```python
from build123d import *

# Parameters (mm, degrees)
SKETCH1_R                  = 12.7
BOSS_EXTRUDE1_DEPTH        = 15.875
SHELL1_T                   = -6.35
SKETCH4_R                  = 1.2446
CUT_EXTRUDE1_DEPTH         = 24.970724332
CUT_EXTRUDE1_DEPTH_BACK    = 24.970724332
SKETCH7_R                  = 7.6962
SKETCH7_R_2                = 6.35
CUT_EXTRUDE2_DEPTH         = 2.3622
TAP_DRILL_FOR_10_32_TAP1_D = 4.0386
CIRPATTERN1_COUNT          = 6


with BuildPart() as part:
    # Sketch1 → Boss-Extrude1 (new body)
    with BuildSketch(Plane.XY):
        Circle(SKETCH1_R)
    extrude(amount=-BOSS_EXTRUDE1_DEPTH)

    # Shell1
    shell1_openings = [part.faces().sort_by_distance(p)[0] for p in [
        (0, 0, -15.875),
    ]]
    offset(amount=SHELL1_T, openings=shell1_openings, kind=Kind.INTERSECTION)

    # Sketch4 → Cut-Extrude1 (cut, two sides)
    with BuildSketch(Plane(origin=(0, 0, 0), x_dir=(0, 0, -1), z_dir=(1, 0, 0))) as cut_extrude1_sk:
        with Locations((9.8425, 0)):
            Circle(SKETCH4_R)
    extrude(amount=CUT_EXTRUDE1_DEPTH, mode=Mode.SUBTRACT)
    extrude(cut_extrude1_sk.sketch, amount=-CUT_EXTRUDE1_DEPTH_BACK, mode=Mode.SUBTRACT)

    # Sketch7 → Cut-Extrude2 (cut)
    with BuildSketch(Plane(origin=(0, 0, -14.605), x_dir=(-1, 0, 0), z_dir=(0, 0, -1))):
        Circle(SKETCH7_R)
        with Locations(Location((0, 0, 0), (0, 0, 180))):
            Circle(SKETCH7_R_2, mode=Mode.SUBTRACT)
    extrude(amount=-CUT_EXTRUDE2_DEPTH, mode=Mode.SUBTRACT)

    # Tap Drill for #10-32 Tap1 (through all)
    with Locations(Plane.XY):
        with Locations((0, 0)):
            Hole(TAP_DRILL_FOR_10_32_TAP1_D / 2)

    # Sketch15 → Tap Drill for #4-40 Tap1 (revolve, cut)
    with BuildSketch(Plane(origin=(-10.16, 0, 0), x_dir=(0, -1, 0), z_dir=(1, 0, 0))):
        Polygon((0, 0), (0, 5.759152758), (1.1303, 5.08), (1.1303, 0), align=None)
    tap_drill_for_4_40_tap1 = revolve(axis=Axis((-10.16, 0, 6.35), (0, 0, -1)), mode=Mode.SUBTRACT)

    # CirPattern1: Tap Drill for #4-40 Tap1 ×6 about axis
    cirpattern1_axis = Axis((0, 0, 0), (0, 0, 1))
    for i in range(1, CIRPATTERN1_COUNT):
        add(tap_drill_for_4_40_tap1.rotate(cirpattern1_axis, i * 360 / CIRPATTERN1_COUNT), mode=Mode.SUBTRACT)


solid = part.part
```
Input: part model. Units: mm. Frame: model coordinates. A direction names the side the tool comes from. Round coordinates to 2 decimals unless told otherwise and drop trailing zeros. Order: outer loops, then holes, each group sorted by start corner. A loop starts at its lowest first (then second) coordinate and runs counter-clockwise, first axis right, second up. Notation, with made-up numbers: (42, -7.75) - (71, -7.75) arc R24 cw to (71, 2.25) - close; hole circle Ø10 at (37.5, 76.5). An arc over 180 degrees is marked (long way). Answer in a Markdown table with one row per item.
Item 1: Section query C-C (y = 5.5). Return the cut outline in (x, z) (3 decimals), then the cut area to 3 significant figures.
Model answer:
| item | result |
|---|---|
| outline | (-11.447, -15.875) - (-3.174, -15.875) - (-3.174, -14.605) - (-5.383, -14.605) - (-5.383, -12.243) - (-3.174, -12.243) - (-3.174, -6.35) - (3.174, -6.35) - (3.174, -12.243) - (5.383, -12.243) - (5.383, -14.605) - (3.174, -14.605) - (3.174, -15.875) - (11.447, -15.875) - (11.447, 0) - (-11.447, 0) - close |
| area | 293 mm² |
Item 2: Reachability of faces 4 (the cylindrical face through (-1.38, -6.2, -15.23)), 5 (the flat face through (0, -3, 0)), 6 (the cylindrical face through (9.057, -0.245, -2.504)), 7 (the flat face through (3, 6, -15.875)), 8 (the cylindrical face through (1.668, -7.513, -13.44)) from +Z, -Z, +X, -X, +Y, -Y: full face, straight path, thin tool, end or side. Return the list, or none.
Model answer:
| item | result |
|---|---|
| face 4 | -Z |
| face 5 | +Z, +X, -X, +Y, -Y |
| face 6 | +Z |
| face 7 | -Z, +X, -X, +Y, -Y |
| face 8 | none |
Item 3: Line query: line 1 (Y direction, x = 0, z = -14.05); line 2 (Z direction, x = -7.25, y = -1.75) (3 decimals); line 3 (X direction, y = 0.25, z = -12.5). Output: solid intervals per line, ascending.
Model answer:
| item | result |
|---|---|
| line 1 | y = -12.7 to -7.7, 7.7 to 12.7 |
| line 2 | z = -15.875 to -14.605, -12.243 to 0 |
| line 3 | x = -12.7 to -7.69, 7.69 to 12.7 |
Item 4: Section query B-B (z = -3). Return the cut outline in (x, y).
Model answer:
| item | result |
|---|---|
| outline | circle Ø25.4 at (0, 0); hole circle Ø2.26 at (-10.16, 0); hole circle Ø2.26 at (-5.08, -8.8); hole circle Ø2.26 at (-5.08, 8.8); hole circle Ø4.04 at (0, 0); hole circle Ø2.26 at (5.08, -8.8); hole circle Ø2.26 at (5.08, 8.8); hole circle Ø2.26 at (10.16, 0) |
Item 5: Pin query (flat end, axial travel): pin 1 (3 mm diameter, centred on x = 1.5, z = -5.5, fed in from -Y); pin 2 (6.5 mm diameter, centred on x = 0, y = 0, fed in from -Z); pin 3 (1 mm diameter, centred on y = -8, z = -2, fed in from +X); pin 4 (2 mm diameter, centred on x = -3, z = -6, fed in from -Y). Return the tip coordinate at first contact, or that it passes through.
Model answer:
| item | result |
|---|---|
| pin 1 | stops at y = -12.7 |
| pin 2 | stops at z = -6.35 |
| pin 3 | stops at x = 10.25 |
| pin 4 | stops at y = -12.54 |
Item 6: Section query A-A (x = 0). Return the cut outline in (y, z) (3 decimals), then the cut area to 3 significant figures.
Model answer:
| item | result |
|---|---|
| outline | (-12.7, -15.875) - (-6.35, -15.875) - (-6.35, -14.605) - (-7.696, -14.605) - (-7.696, -12.243) - (-6.35, -12.243) - (-6.35, -6.35) - (-2.019, -6.35) - (-2.019, 0) - (-12.7, 0) - close; (2.019, -6.35) - (6.35, -6.35) - (6.35, -12.243) - (7.696, -12.243) - (7.696, -14.605) - (6.35, -14.605) - (6.35, -15.875) - (12.7, -15.875) - (12.7, 0) - (2.019, 0) - close |
| area | 250 mm² |
Item 7: Mould query, pull axis Z, two halves, no side actions, for faces 1 (the conical face through (4.885, 8.824, -5.641)), 2 (the cylindrical face through (-6.083, -8.277, -2.504)), 3 (the cylindrical face through (-9.4, 0.1, -8.6)). Classes: released by +Z, released by -Z, zero draft, split by the parting line, or undercut.
Model answer:
| item | result |
|---|---|
| face 1 | released by +Z |
| face 2 | zero draft |
| face 3 | undercut |
Item 8: Section query D-D (z = -9.25). Return the cut outline in (x, y).
Model answer:
| item | result |
|---|---|
| outline | (-12.65, -1.09) arc R12.7 ccw to (12.65, -1.09) - (6.25, -1.09) arc R6.35 cw to (-6.25, -1.09) - close; (-12.65, 1.09) - (-6.25, 1.09) arc R6.35 cw to (6.25, 1.09) - (12.65, 1.09) arc R12.7 ccw to start |
